Answer from the drawing. Dimensions are ordinates in mm from the lowest x, y and z of the part. Coordinates: 2 decimals unless noted, no trailing zeros. Order: outer loops, then holes, each group sorted by start corner. A loop starts at its lowest first (then second) coordinate and runs counter-clockwise, first axis right, second up. Notation, with made-up numbers: M 29,-30 L 63,-30 A14 cw 63,-7 Z; hole C 86.25,62.25 d8. An arc over 180 degrees is marked long. One line per question, with ' | ' between items. Start each with the question number.
1) Given P1, Ø5.5, axis at x = 92.5, y = 10.5, coming from the +Z side; P2, Ø4, axis at x = 54, y = 13.5, coming from the +Z side; P3, Ø1, axis at x = 29, z = 13, coming from the +Y side (1 decimal), each flat-ended and moving along its own axis, determine where each tip first touches the part or whether it passes through.
2) Find section B-B, the plane x = 5. Write down the section's boundary in (y, z) (1 decimal).
3) Find section C-C, the plane z = 8.5. Write down the section's boundary in (x, y), plus the area to 3 significant figures.
4) Consider probe 1 along X at (y, z) = (10, 9); probe 2 along X at (y, z) = (10, 1.5); probe 3 along Y at (x, z) = (93, 11.75). Determine where each line is inside the solid, lowest interval first.
5) Find section A-A, the plane y = 10. Write down the section's boundary in (x, z).
6) Find section D-D, the plane y = 5.75. Write down the section's boundary in (x, z), plus the area to 3 significant figures.
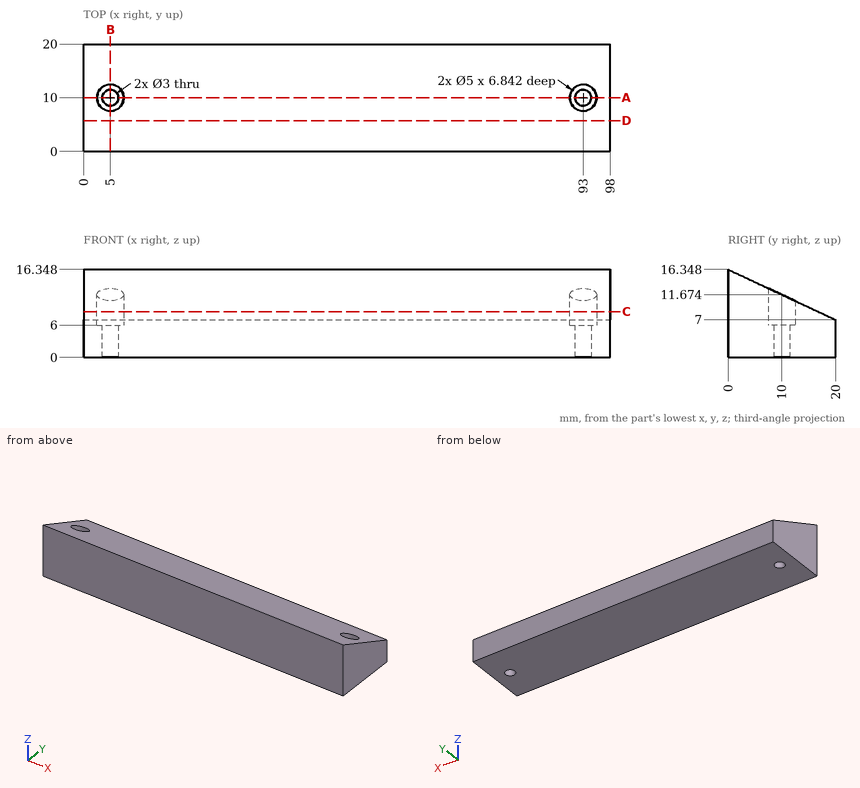
Report:
1) P1: stops at z = 12.67 | P2: stops at z = 10.97 | P3: stops at y = 8.2
2) outline: M 0,0 L 8.5,0 L 8.5,6 L 7.5,6 L 7.5,12.8 L 0,16.3 Z; M 11.5,0 L 20,0 L 20,7 L 12.5,10.5 L 12.5,6 L 11.5,6 Z
3) outline: M 0,0 L 98,0 L 98,16.79 L 0,16.79 Z; hole C 5,10 d5; hole C 93,10 d5 | area: 1,610 mm^2
4) probe 1: x = 0 to 2.5, 7.5 to 90.5, 95.5 to 98 | probe 2: x = 0 to 3.5, 6.5 to 91.5, 94.5 to 98 | probe 3: y = 0 to 7.5
5) outline: M 0,0 L 3.5,0 L 3.5,6 L 2.5,6 L 2.5,11.67 L 0,11.67 Z; M 6.5,0 L 91.5,0 L 91.5,6 L 90.5,6 L 90.5,11.67 L 7.5,11.67 L 7.5,6 L 6.5,6 Z; M 94.5,0 L 98,0 L 98,11.67 L 95.5,11.67 L 95.5,6 L 94.5,6 Z
6) outline: M 0,0 L 98,0 L 98,13.66 L 0,13.66 Z | area: 1,340 mm^2
